```python
from build123d import *

# Parameters (mm, degrees)
F0_W     = 1.5
F0_H     = 31.3
F0_R     = 1.3
F0_W_2   = 79.3
F0_H_2   = 1.5
F1_DEPTH = 4
F0_R_2   = 2.55
F2_DEPTH = 1.6
F0_R_3   = 1.55
F3_DEPTH = 3.45
F4_R     = 1.3
F5_DEPTH = 1
F6_SIZE  = 1
F7_R     = 0.6


with BuildPart() as f1:
    # F0 (on Top) → F1 (new body)
    with BuildSketch(Plane.XY):
        with Locations((-46.25, 0)):
            Rectangle(F0_W, F0_H)
        with BuildLine():
            Line((-45.5, -15.65), (-47, -15.65))
            Line((-47, -15.65), (-47, -20))
            ThreePointArc((-47, -20), (-46.1213203436, -22.1213203436), (-44, -23))
            Line((-44, -23), (-39.65, -23))
            Line((-39.65, -23), (-39.65, -21.5))
            Line((-39.65, -21.5), (-45.5, -21.5))
            Line((-45.5, -21.5), (-45.5, -15.65))
        make_face()
        with BuildLine():
            Line((-41.65, -15.65), (-45.5, -15.65))
            Line((-45.5, -15.65), (-45.5, -21.5))
            Line((-45.5, -21.5), (-39.65, -21.5))
            Line((-39.65, -21.5), (-39.65, -17.65))
            ThreePointArc((-39.65, -17.65), (-40.2357864376, -16.2357864376), (-41.65, -15.65))
        make_face()
        with Locations((-42.95, -18.95)):
            Circle(F0_R, mode=Mode.SUBTRACT)
        with Locations((0, -22.25)):
            Rectangle(F0_W_2, F0_H_2)
        with BuildLine():
            Line((-39.65, 23), (-44, 23))
            ThreePointArc((-44, 23), (-46.1213203436, 22.1213203436), (-47, 20))
            Line((-47, 20), (-47, 15.65))
            Line((-47, 15.65), (-45.5, 15.65))
            Line((-45.5, 15.65), (-45.5, 21.5))
            Line((-45.5, 21.5), (-39.65, 21.5))
            Line((-39.65, 21.5), (-39.65, 23))
        make_face()
        with BuildLine():
            Line((-39.65, 17.65), (-39.65, 21.5))
            Line((-39.65, 21.5), (-45.5, 21.5))
            Line((-45.5, 21.5), (-45.5, 15.65))
            Line((-45.5, 15.65), (-41.65, 15.65))
            ThreePointArc((-41.65, 15.65), (-40.2357864376, 16.2357864376), (-39.65, 17.65))
        make_face()
        with Locations((-42.95, 18.95)):
            Circle(F0_R, mode=Mode.SUBTRACT)
        with Locations((0, 22.25)):
            Rectangle(F0_W_2, F0_H_2)
        with BuildLine():
            Line((44, 23), (39.65, 23))
            Line((39.65, 23), (39.65, 21.5))
            Line((39.65, 21.5), (45.5, 21.5))
            Line((45.5, 21.5), (45.5, 15.65))
            Line((45.5, 15.65), (47, 15.65))
            Line((47, 15.65), (47, 20))
            ThreePointArc((47, 20), (46.1213203436, 22.1213203436), (44, 23))
        make_face()
        with BuildLine():
            Line((45.5, 21.5), (39.65, 21.5))
            Line((39.65, 21.5), (39.65, 17.65))
            ThreePointArc((39.65, 17.65), (40.2357864376, 16.2357864376), (41.65, 15.65))
            Line((41.65, 15.65), (45.5, 15.65))
            Line((45.5, 15.65), (45.5, 21.5))
        make_face()
        with Locations((42.95, 18.95)):
            Circle(F0_R, mode=Mode.SUBTRACT)
        with BuildLine():
            Line((45.5, -21.5), (45.5, -15.65))
            Line((45.5, -15.65), (41.65, -15.65))
            ThreePointArc((41.65, -15.65), (40.2357864376, -16.2357864376), (39.65, -17.65))
            Line((39.65, -17.65), (39.65, -21.5))
            Line((39.65, -21.5), (45.5, -21.5))
        make_face()
        with Locations((42.95, -18.95)):
            Circle(F0_R, mode=Mode.SUBTRACT)
        with BuildLine():
            Line((47, -20), (47, -15.65))
            Line((47, -15.65), (45.5, -15.65))
            Line((45.5, -15.65), (45.5, -21.5))
            Line((45.5, -21.5), (39.65, -21.5))
            Line((39.65, -21.5), (39.65, -23))
            Line((39.65, -23), (44, -23))
            ThreePointArc((44, -23), (46.1213203436, -22.1213203436), (47, -20))
        make_face()
        with Locations((46.25, 0)):
            Rectangle(F0_W, F0_H)
    extrude(amount=F1_DEPTH)

    # F0 (on Top) → F2 (join)
    with BuildSketch(Plane.XY):
        with BuildLine():
            Line((39.65, 21.5), (-39.65, 21.5))
            Line((-39.65, 21.5), (-39.65, 17.65))
            ThreePointArc((-39.65, 17.65), (-40.2357864376, 16.2357864376), (-41.65, 15.65))
            Line((-41.65, 15.65), (-45.5, 15.65))
            Line((-45.5, 15.65), (-45.5, -15.65))
            Line((-45.5, -15.65), (-41.65, -15.65))
            ThreePointArc((-41.65, -15.65), (-40.2357864376, -16.2357864376), (-39.65, -17.65))
            Line((-39.65, -17.65), (-39.65, -21.5))
            Line((-39.65, -21.5), (39.65, -21.5))
            Line((39.65, -21.5), (39.65, -17.65))
            ThreePointArc((39.65, -17.65), (40.2357864376, -16.2357864376), (41.65, -15.65))
            Line((41.65, -15.65), (45.5, -15.65))
            Line((45.5, -15.65), (45.5, 15.65))
            Line((45.5, 15.65), (41.65, 15.65))
            ThreePointArc((41.65, 15.65), (40.2357864376, 16.2357864376), (39.65, 17.65))
            Line((39.65, 17.65), (39.65, 21.5))
        make_face()
        with Locations((-39.75, 0)):
            Circle(F0_R_2, mode=Mode.SUBTRACT)
        with BuildLine():
            ThreePointArc((-37, 18), (-36.4142135624, 19.4142135624), (-35, 20))
            Line((-35, 20), (35, 20))
            ThreePointArc((35, 20), (36.4142135624, 19.4142135624), (37, 18))
            Line((37, 18), (37, -18))
            ThreePointArc((37, -18), (36.4142135624, -19.4142135624), (35, -20))
            Line((35, -20), (-35, -20))
            ThreePointArc((-35, -20), (-36.4142135624, -19.4142135624), (-37, -18))
            Line((-37, -18), (-37, 18))
        make_face(mode=Mode.SUBTRACT)
        with Locations((39.75, 0)):
            Circle(F0_R_2, mode=Mode.SUBTRACT)
    extrude(amount=F2_DEPTH)

    # F0 (on Top) → F3 (join)
    with BuildSketch(Plane.XY):
        with Locations((-39.75, 0)):
            Circle(F0_R_2)
        with Locations((-39.75, 0)):
            Circle(F0_R_3, mode=Mode.SUBTRACT)
        with Locations((39.75, 0)):
            Circle(F0_R_2)
        with Locations((39.75, 0)):
            Circle(F0_R_3, mode=Mode.SUBTRACT)
    extrude(amount=F3_DEPTH)

    # F4 (on face) → F5 (cut)
    with BuildSketch(Plane.XY.offset(4)):
        with BuildLine():
            Line((-45.5, 19.5), (-45.5, 15.65))
            Line((-45.5, 15.65), (-41.65, 15.65))
            ThreePointArc((-41.65, 15.65), (-40.2357864376, 16.2357864376), (-39.65, 17.65))
            Line((-39.65, 17.65), (-39.65, 21.5))
            Line((-39.65, 21.5), (-43.5, 21.5))
            ThreePointArc((-43.5, 21.5), (-44.9142135624, 20.9142135624), (-45.5, 19.5))
        make_face()
        with Locations((-42.95, 18.95)):
            Circle(F4_R, mode=Mode.SUBTRACT)
        with BuildLine():
            Line((-41.65, -15.65), (-45.5, -15.65))
            Line((-45.5, -15.65), (-45.5, -19.5))
            ThreePointArc((-45.5, -19.5), (-44.9142135624, -20.9142135624), (-43.5, -21.5))
            Line((-43.5, -21.5), (-39.65, -21.5))
            Line((-39.65, -21.5), (-39.65, -17.65))
            ThreePointArc((-39.65, -17.65), (-40.2357864376, -16.2357864376), (-41.65, -15.65))
        make_face()
        with Locations((-42.95, -18.95)):
            Circle(F4_R, mode=Mode.SUBTRACT)
        with BuildLine():
            Line((39.65, -17.65), (39.65, -21.5))
            Line((39.65, -21.5), (43.5, -21.5))
            ThreePointArc((43.5, -21.5), (44.9142135624, -20.9142135624), (45.5, -19.5))
            Line((45.5, -19.5), (45.5, -15.65))
            Line((45.5, -15.65), (41.65, -15.65))
            ThreePointArc((41.65, -15.65), (40.2357864376, -16.2357864376), (39.65, -17.65))
        make_face()
        with Locations((42.95, -18.95)):
            Circle(F4_R, mode=Mode.SUBTRACT)
        with BuildLine():
            Line((43.5, 21.5), (39.65, 21.5))
            Line((39.65, 21.5), (39.65, 17.65))
            ThreePointArc((39.65, 17.65), (40.2357864376, 16.2357864376), (41.65, 15.65))
            Line((41.65, 15.65), (45.5, 15.65))
            Line((45.5, 15.65), (45.5, 19.5))
            ThreePointArc((45.5, 19.5), (44.9142135624, 20.9142135624), (43.5, 21.5))
        make_face()
        with Locations((42.95, 18.95)):
            Circle(F4_R, mode=Mode.SUBTRACT)
    extrude(amount=-F5_DEPTH, mode=Mode.SUBTRACT)

    # F6
    f6_edges = [f1.edges().sort_by_distance(p)[0] for p in [
        (41.65, 18.95, 0),
        (41.65, -18.95, 0),
        (-44.25, -18.95, 0),
        (-44.25, 18.95, 0),
    ]]
    chamfer(f6_edges, length=F6_SIZE)

    # F7
    f7_edges = [f1.edges().sort_by_distance(p)[0] for p in [
        (37.2, 0, 3.45),
        (-42.3, 0, 3.45),
    ]]
    fillet(f7_edges, radius=F7_R)


solid = f1.part
```
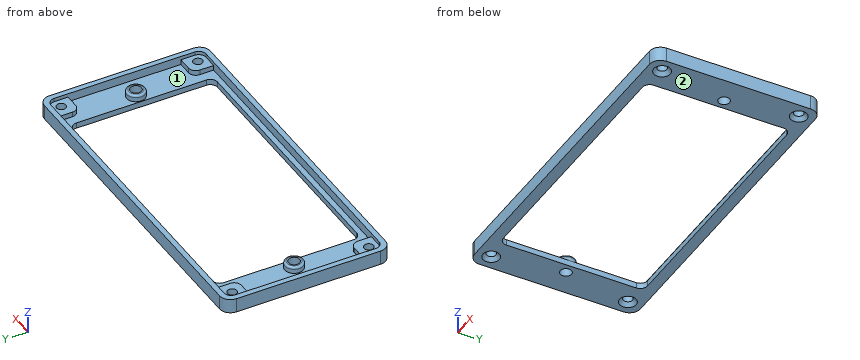
Verification items for the finished model (mm, model axes). Face numbers are marked on the shaded views. Coordinates: 2 decimals unless noted, no trailing zeros. Loops run counter-clockwise (first coordinate to the right, second up) from the corner with the lowest first, then second, coordinate; pieces in that order, holes last. Notation, with made-up numbers: (63.5, -24.75) - (110.5, -24.75) arc R19 cw to (110.5, 11.25) - close; hole circle Ø2 at (83, 25). An arc over 180 degrees is marked (long way). Return JSON: item names as keys, results as strings.
1. Go/stop test with flat-tipped pins: pin 1 (1.8 mm diameter, centred on x = 41.5, y = -18, fed in from +Z); pin 2 (3 mm diameter, centred on x = 40.5, y = -1, fed in from +Z); pin 3 (3 mm diameter, centred on x = 42.95, y = 18.95, fed in from -Z). Record where each tip stops, or that it passes through.
Established:
{"pin 1": "stops at z = 3", "pin 2": "stops at z = 3.45", "pin 3": "stops at z = 0.8"}
2. Section check A-A, the plane x = 7.5. Record the boundary of the cut face in (y, z), then the cut area to 3 significant figures.
Established:
{"outline": "(-23, 0) - (-20, 0) - (-20, 1.6) - (-21.5, 1.6) - (-21.5, 4) - (-23, 4) - close; (20, 0) - (23, 0) - (23, 4) - (21.5, 4) - (21.5, 1.6) - (20, 1.6) - close", "area": "16.8 mm2"}
3. Mould release check, pull along Y, two halves, no side actions. Record for the marked faces 1 and 2: +Y half, -Y half, draft (parallel to the pull), parting line (faces both ways), or undercut.
Established:
{"face 1": "undercut", "face 2": "draft"}
4. Section check B-B, the plane y = -13.5. Record the boundary of the cut face in (x, z).
Established:
{"outline": "(-47, 0) - (-37, 0) - (-37, 1.6) - (-45.5, 1.6) - (-45.5, 4) - (-47, 4) - close; (37, 0) - (47, 0) - (47, 4) - (45.5, 4) - (45.5, 1.6) - (37, 1.6) - close"}
5. Thickness scan on L1, parallel to X at y = -11, z = 1.5; L2, parallel to Y at x = -42.95, z = 2; L3, parallel to X at y = -17, z = 3.15. Record the ranges inside material, lowest first.
Established:
{"L1": "x = -47 to -37, 37 to 47", "L2": "y = -23 to -20.25, -17.65 to -15.65, 15.65 to 17.65, 20.25 to 23", "L3": "x = -47 to -45.5, 45.5 to 47"}
